The drawing under review shows one solid part. Ordinate dimensions are in mm from its lowest x, y, z. Round coordinates to 2 decimals unless told otherwise and drop trailing zeros. Write each loop counter-clockwise with the first axis right and the second up, starting at its lowest first coordinate (ties: lowest second). Pieces come first, ordered by that corner, then holes. Notation, with made-up numbers: (-31, 35.25) -> (-16, 35.25) arc R12 ccw to (-16, 40.25) -> close; hole circle Ø6 at (46.5, 86). An arc over 180 degrees is marked (long way). Answer in a Markdown table with one row per item.
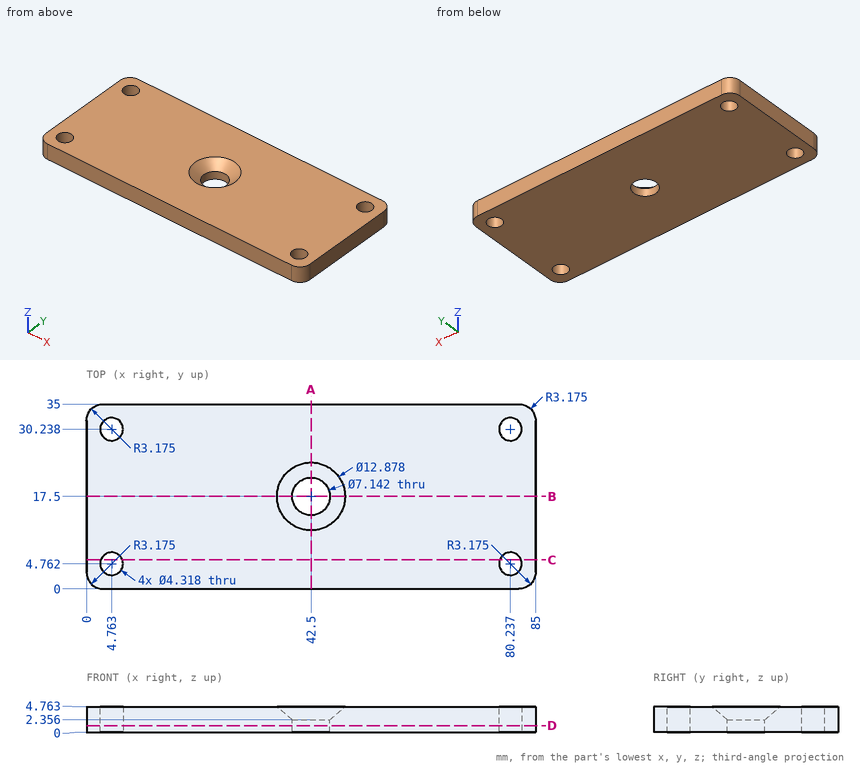
1) Consider section B-B on y = 17.5. State the section outline as (x, z) points.
Solved:
| item | result |
|---|---|
| outline | (0, 0) -> (38.93, 0) -> (38.93, 2.36) -> (36.06, 4.76) -> (0, 4.76) -> close; (46.07, 0) -> (85, 0) -> (85, 4.76) -> (48.94, 4.76) -> (46.07, 2.36) -> close |
2) Consider section A-A on x = 42.5. State the section outline as (y, z) points.
Solved:
| item | result |
|---|---|
| outline | (0, 0) -> (13.93, 0) -> (13.93, 2.36) -> (11.06, 4.76) -> (0, 4.76) -> close; (21.07, 0) -> (35, 0) -> (35, 4.76) -> (23.94, 4.76) -> (21.07, 2.36) -> close |
3) Clearance check with flat-ended pins moving along their axes: pin 1 Ø5.5 at (x, y) = (4.76, 30.24) entering from -Z; pin 2 Ø9.5 at (x, y) = (42.5, 17.5) entering from +Z (1 decimal). State where each tip first meets the part, or that it passes through.
Solved:
| item | result |
|---|---|
| pin 1 | z = 0 |
| pin 2 | z = 3.3 |
4) Consider section C-C on y = 5.5. State the section outline as (x, z) points.
Solved:
| item | result |
|---|---|
| outline | (0, 0) -> (2.73, 0) -> (2.73, 4.76) -> (0, 4.76) -> close; (6.79, 0) -> (78.21, 0) -> (78.21, 4.76) -> (6.79, 4.76) -> close; (82.27, 0) -> (85, 0) -> (85, 4.76) -> (82.27, 4.76) -> close |
5) For line 1 (X direction, y = 3, z = 0.7) (1 decimal); line 2 (Y direction, x = 3, z = 3.5) (1 decimal); line 3 (Y direction, x = 43, z = 0.55) (1 decimal), list the stretches that pass through material, from the lowest coordinate up. Write a range as [from, to].
Solved:
| item | result |
|---|---|
| line 1 | [0, 3.5], [6, 79], [81.5, 85] |
| line 2 | [0, 3.5], [6, 29], [31.5, 35] |
| line 3 | [0, 14], [21, 35] |
6) Consider section D-D on z = 1.2. State how many separate pieces and enclosed holes the cut face has, then the cut area to 3 significant figures.
Solved:
| item | result |
|---|---|
| separate pieces | 1 |
| enclosed holes | 5 |
| area | 2,870 mm² |
